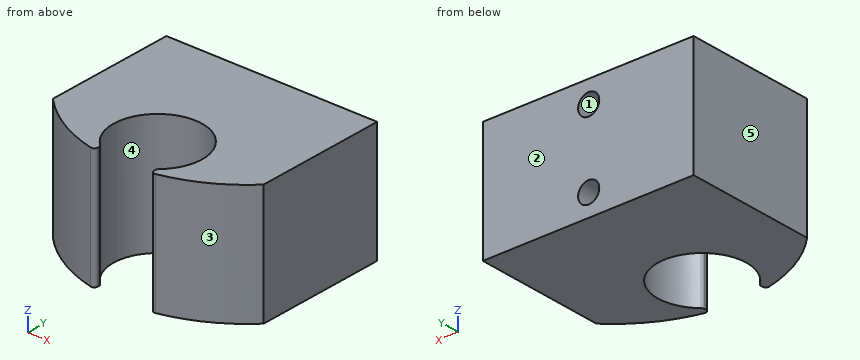
from build123d import *

# Parameters (mm, degrees)
BOSS_EXTRUDE1_START = -8.5
BOSS_EXTRUDE1_DEPTH = 17
CUT_EXTRUDE2_DEPTH  = 30.420443572
FILLET1_R           = 0.5
FILLET2_R           = 0.5
FILLET3_R           = 0.5
FILLET4_R           = 0.5
SKETCH3_R           = 1.5
CUT_EXTRUDE3_DEPTH  = 5


# Read off the part's stored shape, not the designer's step: Boss-Extrude1
with BuildPart() as part:
    # Boss-Extrude1 outline → Boss-Extrude1 (new body)
    with BuildSketch(Plane.XY.offset(BOSS_EXTRUDE1_START)):
        with BuildLine():
            ThreePointArc((-0.026346322, -6.254944514), (0.013173118, 6.254986128), (0, -6.255))
            ThreePointArc((0, -6.255), (8.130777353, -4.640165574), (15, 0))
            Line((15, 0), (15, 18.75))
            Line((15, 18.75), (-14.876085662, 18.75))
            Line((-14.876085662, 18.75), (-14.876085662, 0))
            ThreePointArc((-14.876085662, 0), (-8.076154016, -4.611125189), (-0.026346322, -6.254944514))
        make_face()
    extrude(amount=BOSS_EXTRUDE1_DEPTH)

    # Sketch2 → Cut-Extrude2 (cut, through all)
    with BuildSketch(Plane.XY.offset(8.5)):
        Polygon((4, 0), (0, 0), (-4, 0), (-4, -9.216790773), (4, -9.216790773), align=None)
    extrude(amount=-CUT_EXTRUDE2_DEPTH, mode=Mode.SUBTRACT)

    # Fillet1
    fillet1_edges = [part.edges().sort_by_distance(p)[0] for p in [
        (4, -4.808848585, 0),
    ]]
    fillet(fillet1_edges, radius=FILLET1_R)

    # Fillet2
    fillet2_edges = [part.edges().sort_by_distance(p)[0] for p in [
        (4, -5.881926017, 0),
    ]]
    fillet(fillet2_edges, radius=FILLET2_R)

    # Fillet3
    fillet3_edges = [part.edges().sort_by_distance(p)[0] for p in [
        (-4, -4.808848645, 0),
    ]]
    fillet(fillet3_edges, radius=FILLET3_R)

    # Fillet4
    fillet4_edges = [part.edges().sort_by_distance(p)[0] for p in [
        (-4, -5.857856611, 0),
    ]]
    fillet(fillet4_edges, radius=FILLET4_R)

    # Sketch3 → Cut-Extrude3 (cut)
    with BuildSketch(Plane(origin=(0, 18.75, 0), x_dir=(1, 0, 0), z_dir=(0, 1, 0))):
        with Locations(Location((0, -5.375, 0), (0, 0, 270))):
            Circle(SKETCH3_R)
        with Locations(Location((0, 5.375, 0), (0, 0, 270))):
            Circle(SKETCH3_R)
    extrude(amount=-CUT_EXTRUDE3_DEPTH, mode=Mode.SUBTRACT)


solid = part.part
Can you work these out from the model? Positions are in its coordinate system, mm. Face numbers are marked on the shaded views. A direction names the side the tool comes from. Give positions to 0.01 mm unless a question says otherwise; leave off trailing zeros. Order: outer loops, then holes, each group sorted by start corner. A loop starts at its lowest first (then second) coordinate and runs counter-clockwise, first axis right, second up. Notation, with made-up numbers: M 71.5,37.5 L 94.5,37.5 A9 cw 94.5,50.5 Z; hole C -2.5,65.5 d9. An arc over 180 degrees is marked long. Use a Markdown table: item, result. Add a question column.
Item 1: Suppose I cut it at B-B (y = 3.25). List the corners of the cut face in (x, z) for me, then the cut area to 3 significant figures.
Item 2: If I drill on L1, parallel to X at y = 4.75, z = -6; L2, parallel to X at y = -3.25, z = -3; L3, parallel to Y at x = 0, z = 0.5 (3 decimals), over which ranges is the centre line in solid material (lowest first)? Write a range as [from, to].
Item 3: Suppose I cut it at C-C (x = 0). List the corners of the cut face in (y, z) for me (3 decimals).
Item 4: Suppose I cut it at A-A (x = -5). List the corners of the cut face in (y, z) for me, then the cut area to 3 significant figures.
Item 5: We'd pull the mould along X, two halves only. Please class the marked faces 3, 4 and 5: +X half, -X half, draft (parallel to the pull), parting line (faces both ways), or undercut.
Item 6: Will these pins go through, and if not, where does the flat tip stop? pin 1 (1.8 mm diameter, centred on x = 0, z = 5.375, fed in from +Y); pin 2 (11.5 mm diameter, centred on x = 0, y = 0, fed in from +Z).
Item 7: For the marked faces 1 and 2, which set-ups out of +Z, -Z, +X, -X, +Y, -Y let a thin tool reach every point of the face, with its end or its side?
Item 8: Suppose I cut it at D-D (z = 3.25). List the corners of the cut face in (x, y) for me (3 decimals).
Answer sheet:
| question | item | result |
|---|---|---|
| 1 | outline | M -14.88,-8.5 L -5.34,-8.5 L -5.34,8.5 L -14.88,8.5 Z; M 5.34,-8.5 L 15,-8.5 L 15,8.5 L 5.34,8.5 Z |
| 1 | area | 326 mm² |
| 2 | L1 | x = [-14.88, -4.07], [4.07, 15] |
| 2 | L2 | x = [-10.75, -5.34], [5.34, 10.88] |
| 2 | L3 | y = [6.255, 18.75] |
| 3 | outline | M 6.255,-8.5 L 18.75,-8.5 L 18.75,-6.875 L 13.75,-6.875 L 13.75,-3.875 L 18.75,-3.875 L 18.75,3.875 L 13.75,3.875 L 13.75,6.875 L 18.75,6.875 L 18.75,8.5 L 6.255,8.5 Z |
| 4 | outline | M -5.63,-8.5 L -3.76,-8.5 L -3.76,8.5 L -5.63,8.5 Z; M 3.76,-8.5 L 18.75,-8.5 L 18.75,8.5 L 3.76,8.5 Z |
| 4 | area | 287 mm² |
| 5 | face 3 | +X half |
| 5 | face 4 | undercut |
| 5 | face 5 | -X half |
| 6 | pin 1 | stops at y = 13.75 |
| 6 | pin 2 | passes through |
| 7 | face 1 | +Y |
| 7 | face 2 | +Z, -Z, +X, -X, +Y |
| 8 | outline | M -14.876,0 A20.965 ccw -4.611,-5.728 A0.5 ccw -4,-5.24 L -4,-5.038 A0.5 ccw -4.167,-4.665 A6.255 cw long 4.167,-4.665 A0.5 ccw 4,-5.038 L 4,-5.268 A0.5 ccw 4.608,-5.756 A20.964 ccw 15,0 L 15,18.75 L -14.876,18.75 Z |
